Verification items for the finished model (mm, model axes). Round coordinates to 2 decimals unless told otherwise and drop trailing zeros. Write each loop counter-clockwise with the first axis right and the second up, starting at its lowest first coordinate (ties: lowest second). Pieces come first, ordered by that corner, then holes. Notation, with made-up numbers: (-19.75, -24.5) -> (-8.75, -24.5) arc R27 cw to (-8.75, 3.5) -> close; hole circle Ø9 at (-27, 82). An arc over 180 degrees is marked (long way). Answer as a JSON object with one key per item and string values. Group by question number.
(1) Scan lines: L1, parallel to Z at x = 1.9, y = 60; L2, parallel to Z at x = 2.1, y = 31; L3, parallel to Z at x = 1.15, y = -43. Record each from-to range of solid material in increasing order. Write a range as from..to.
(2) Sectioned sample at B-B on x = 1.65. Count the separate pieces of the cut face and the enclosed holes in it, and give its area (3 significant figures).
(3) Draft check along Z on faces 1 (the face through (1.268, 0.813, -51.518)), 2 (the face through (1.27, 37.68, 1.63)), 3 (the face through (2.5, 1, 3)). Enter one of: released by +Z, released by -Z, zero draft, split by the parting line, or undercut.
(4) Sectioned sample at A-A on z = -165. Record the cut outline in (x, y), and give its area (4 significant figures).
(5) Gauge pin test, flat ends, axial feed: pin 1 Ø1.2 at (x, y) = (0.5, 81) entering from +Z; pin 2 Ø0.8 at (x, y) = (1, -81.5) entering from -Z; pin 3 Ø1.5 at (x, z) = (0.5, -31) entering from -Y. Record the tip position at first contact, or that the pin passes through.
```python
from build123d import *

# Parameters (mm, degrees)
BOSS_EXTRUDE1_DEPTH = 2.5
SKETCH2_R           = 2.5
SKETCH2_R_2         = 2
SKETCH2_R_3         = 18.5
SKETCH2_R_4         = 28.5
SKETCH2_R_5         = 7.5
SKETCH2_W           = 2.5
SKETCH2_H           = 29.5
CUT_EXTRUDE1_DEPTH  = 2.5


with BuildPart() as part:
    # Sketch1 → Boss-Extrude1 (new body)
    with BuildSketch(Plane(origin=(0, 0, 0), x_dir=(0, 0, -1), z_dir=(1, 0, 0))):
        Polygon((-245, -80), (-148.333333333, -80), (-148.333333333, -82.5), (-48.333333333, -82.5), (-48.333333333, -80), (48.333333333, -80), (48.333333333, -82.5), (148.333333333, -82.5), (148.333333333, -80), (245, -80), (245, 80), (148.333333333, 80), (148.333333333, 82.5), (48.333333333, 82.5), (48.333333333, 80), (-48.333333333, 80), (-48.333333333, 82.5), (-148.333333333, 82.5), (-148.333333333, 80), (-245, 80), align=None)
    extrude(amount=BOSS_EXTRUDE1_DEPTH)

    # Sketch2 → Cut-Extrude1 (cut)
    with BuildSketch(Plane(origin=(2.5, 0, 0), x_dir=(0, 0, -1), z_dir=(1, 0, 0))):
        with Locations((-128.333333333, 61)):
            Circle(SKETCH2_R)
        with Locations((128.333333333, 61)):
            Circle(SKETCH2_R)
        with Locations((128.333333333, -61)):
            Circle(SKETCH2_R)
        with Locations((-128.333333333, -61)):
            Circle(SKETCH2_R)
        with Locations((-223.5, 32.5)):
            Circle(SKETCH2_R)
        with Locations((-223.5, -32.5)):
            Circle(SKETCH2_R)
        with Locations((223.5, 32.5)):
            Circle(SKETCH2_R)
        with Locations((223.5, -32.5)):
            Circle(SKETCH2_R)
        with Locations((-85, 0)):
            Circle(SKETCH2_R_2)
        with Locations((-45, 0)):
            Circle(SKETCH2_R_2)
        with Locations((70, 0)):
            Circle(SKETCH2_R_3)
        with Locations((51.85, 18.15)):
            Circle(SKETCH2_R_2)
        with Locations((51.85, -18.15)):
            Circle(SKETCH2_R_2)
        with Locations((88.15, -18.15)):
            Circle(SKETCH2_R_2)
        with Locations((88.15, 18.15)):
            Circle(SKETCH2_R_2)
        with Locations((-190, -25)):
            Circle(SKETCH2_R)
        with Locations((-165, 0)):
            Circle(SKETCH2_R_4)
        with Locations((-140, -25)):
            Circle(SKETCH2_R)
        with Locations((-140, 25)):
            Circle(SKETCH2_R)
        with Locations((-190, 25)):
            Circle(SKETCH2_R)
        with Locations((165, 0)):
            Circle(SKETCH2_R_4)
        with Locations((190, -25)):
            Circle(SKETCH2_R)
        with Locations((140, -25)):
            Circle(SKETCH2_R)
        with Locations((140, 25)):
            Circle(SKETCH2_R)
        with Locations((190, 25)):
            Circle(SKETCH2_R)
        with Locations((0, 15)):
            Circle(SKETCH2_R_5)
        with Locations((0, -15)):
            Circle(SKETCH2_R_5)
        with Locations((0, 45)):
            Circle(SKETCH2_R_5)
        with Locations((0, -45)):
            Circle(SKETCH2_R_5)
        with Locations((-243.75, 32.5)):
            Rectangle(SKETCH2_W, SKETCH2_H)
        with Locations((-243.75, -32.5)):
            Rectangle(SKETCH2_W, SKETCH2_H)
        with Locations((243.75, -32.5)):
            Rectangle(SKETCH2_W, SKETCH2_H)
        with Locations((243.75, 32.5)):
            Rectangle(SKETCH2_W, SKETCH2_H)
        Polygon((-73.5, 9.5), (-78.5, 4.5), (-78.5, -9.5), (-51.5, -9.5), (-51.5, 4.5), (-56.5, 9.5), align=None)
    extrude(amount=-CUT_EXTRUDE1_DEPTH, mode=Mode.SUBTRACT)


solid = part.part
```
Computed values:
{
 "1": {"L1": "-245..-130.62, -126.04..126.04, 130.62..245", "L2": "-242.5..-225.5, -221.5..221.5, 225.5..242.5", "L3": "-242.5..-7.23, 7.23..242.5"},
 "2": {"separate pieces": "1", "enclosed holes": "30", "area": "71,300 mm2"},
 "3": {"face 1": "undercut", "face 2": "undercut", "face 3": "zero draft"},
 "4": {"outline": "(0, -80) -> (2.5, -80) -> (2.5, -28.5) -> (0, -28.5) -> close; (0, 28.5) -> (2.5, 28.5) -> (2.5, 80) -> (0, 80) -> close", "area": "257.5 mm2"},
 "5": {"pin 1": "z = 148.33", "pin 2": "z = -148.33", "pin 3": "y = -80"}
}
